The model under review builds one solid part; all positions refer to its coordinate system, in mm. A direction names the side the tool comes from. Give positions to 0.01 mm unless a question says otherwise; leave off trailing zeros. Write each loop counter-clockwise with the first axis right and the second up, starting at its lowest first coordinate (ties: lowest second). Pieces come first, ordered by that corner, then holes. Notation, with made-up numbers: M 11.25,75.25 L 18.25,75.25 A26 ccw 18.25,104.25 Z; hole C 56.5,1.25 d8. An arc over 180 degrees is marked long. Write item = value, one per line. Start each with the question number.
```python
from build123d import *

# Parameters (mm, degrees)
SKETCH_1_R               = 8.75
EXTRUDE_1_DEPTH          = 1
EXTRUDE_2_DEPTH          = 1
SKETCH_3_R               = 2.5
CUT_EXTRUDE_1_DEPTH      = 15.091220671
PATTERN_CIRCULAR_1_COUNT = 20
FILLET_1_R               = 0.25


with BuildPart() as part:
    # 草图1 → 凸台-拉伸1 (new body)
    with BuildSketch(Plane(origin=(0, 0, 0), x_dir=(1, 0, 0), z_dir=(0, 1, 0))):
        with Locations(Location((0, 0, 0), (0, 0, 270))):
            Circle(SKETCH_1_R)
    extrude(amount=-EXTRUDE_1_DEPTH)

    # 草图2 → 凸台-拉伸2 (add)
    with BuildSketch(Plane(origin=(0, 0, 0), x_dir=(1, 0, 0), z_dir=(0, 1, 0))):
        with BuildLine():
            Line((-0.765280386, -10.175), (-0.65625, -8.72535592))
            ThreePointArc((-0.65625, -8.72535592), (0, -8.75), (0.65625, -8.72535592))
            Line((0.65625, -8.72535592), (0.765280386, -10.175))
            ThreePointArc((0.765280386, -10.175), (0, -11), (-0.765280386, -10.175))
        make_face()
    extrude_2 = extrude(amount=-EXTRUDE_2_DEPTH)

    # 草图3 → 切除-拉伸1 (cut, through all)
    with BuildSketch(Plane(origin=(0, 0, 0), x_dir=(1, 0, 0), z_dir=(0, 1, 0))):
        with Locations(Location((0, 0, 0), (0, 0, 270))):
            Circle(SKETCH_3_R)
    extrude(amount=-CUT_EXTRUDE_1_DEPTH, mode=Mode.SUBTRACT)

    # 阵列(圆周)1: 凸台-拉伸2 ×20 about axis
    pattern_circular_1_axis = Axis((0, 0, 0), (0, 1, 0))
    for i in range(1, PATTERN_CIRCULAR_1_COUNT):
        add(extrude_2.rotate(pattern_circular_1_axis, i * 360 / PATTERN_CIRCULAR_1_COUNT))

    # 圆角1
    fillet_1_edges = [part.edges().sort_by_distance(p)[0] for p in [
        (3.3204141, -0.5, -8.095514203),
        (2.072152423, -0.5, -8.501099008),
        (0.65625, -0.5, -8.72535592),
        (-0.65625, -0.5, -8.72535592),
        (-2.072152423, -0.5, -8.501099008),
        (-3.3204141, -0.5, -8.095514203),
        (-4.597718128, -0.5, -7.444695293),
        (-5.659552934, -0.5, -6.67322715),
        (-6.67322715, -0.5, -5.659552934),
        (-7.444695293, -0.5, -4.597718128),
        (-8.095514203, -0.5, -3.3204141),
        (-8.501099008, -0.5, -2.072152423),
        (-8.72535592, -0.5, -0.65625),
        (-8.72535592, -0.5, 0.65625),
        (-8.501099008, -0.5, 2.072152423),
        (-8.095514203, -0.5, 3.3204141),
        (-7.444695293, -0.5, 4.597718128),
        (-6.67322715, -0.5, 5.659552934),
        (-5.659552934, -0.5, 6.67322715),
        (-4.597718128, -0.5, 7.444695293),
        (-3.3204141, -0.5, 8.095514203),
        (-2.072152423, -0.5, 8.501099008),
        (2.072152423, -0.5, 8.501099008),
        (3.3204141, -0.5, 8.095514203),
        (4.597718128, -0.5, 7.444695293),
        (5.659552934, -0.5, 6.67322715),
        (6.67322715, -0.5, 5.659552934),
        (7.444695293, -0.5, 4.597718128),
        (8.095514203, -0.5, 3.3204141),
        (8.501099008, -0.5, 2.072152423),
        (8.72535592, -0.5, 0.65625),
        (8.72535592, -0.5, -0.65625),
        (-0.65625, -0.5, 8.72535592),
        (0.65625, -0.5, 8.72535592),
        (8.501099008, -0.5, -2.072152423),
        (8.095514203, -0.5, -3.3204141),
        (7.444695293, -0.5, -4.597718128),
        (6.67322715, -0.5, -5.659552934),
        (5.659552934, -0.5, -6.67322715),
        (4.597718128, -0.5, -7.444695293),
    ]]
    fillet(fillet_1_edges, radius=FILLET_1_R)


solid = part.part
```
Item 1: We need section D-D, the plane x = 5. Write out the cut boundary in (y, z), and give its area (3 significant figures).
Item 2: For faces 5 (the flat face through (5.04, -0.49, -8.16)), 6 (the flat face through (9.32, -0.49, 2.27)), 7 (the flat face through (-9.58, -0.49, -0.72)), 8 (the flat face through (-2.27, -0.49, 9.32)), list the 3-axis set-ups (+Z, -Z, +X, -X, +Y, -Y) from which the entire face can be reached by the end or side of a thin tool; tool diameter is ignored.
Item 3: We need section A-A, the plane z = 0. Write out the cut boundary in (x, y).
Item 4: We need section C-C, the plane z = 2.75. Write out the cut boundary in (x, y), and give its area (3 significant figures).
Item 5: We need section B-B, the plane x = 0. Write out the cut boundary in (y, z), and give its area (3 significant figures).
Item 6: To check wall thickness, follow probe 1 along Z at (x, y) = (-8.25, -0.35); probe 2 along Z at (x, y) = (6.5, -0.3); probe 3 along X at (y, z) = (-0.3, 8.5). State the ranges of each line that lie inside material, in increasing order. Write a range as [from, to].
Item 7: The part is to be moulded in two halves that separate along X. For faces 1 (the flat face through (-3.64, -0.49, -8.87)), 2 (the flat face through (-9.32, -0.49, -2.27)), 3 (the flat face through (5.05, -0.49, 8.18)), 4 (the cylindrical face through (8.643, -0.493, -1.362)), say which applies: released by +X, released by -X, zero draft, split by the parting line, or undercut.
Worked out:
q1.outline = M -1,-8.1 L 0,-8.1 L 0,8.1 L -1,8.1 Z
q1.area = 16.2 mm²
q2.face_5 = -Z, +Y, -Y
q2.face_6 = +X, +Y, -Y
q2.face_7 = +Y, -Y
q2.face_8 = +Z, +Y, -Y
q3.outline = M -11,-1 L -2.5,-1 L -2.5,0 L -11,0 Z; M 2.5,-1 L 11,-1 L 11,0 L 2.5,0 Z
q4.outline = M -10.38,-1 L 10.38,-1 L 10.38,0 L -10.38,0 Z
q4.area = 20.8 mm²
q5.outline = M -1,-11 L 0,-11 L 0,-2.5 L -1,-2.5 Z; M -1,2.5 L 0,2.5 L 0,11 L -1,11 Z
q5.area = 17.0 mm²
q6.probe_1 = [-6.78, -5.1], [-3.4, 3.4], [5.1, 6.78]
q6.probe_2 = [-8.87, -7.66], [-5.86, 5.86], [7.66, 8.87]
q6.probe_3 = [-6.75, -5.25], [-3.49, 3.49], [5.25, 6.75]
q7.face_1 = undercut
q7.face_2 = released by -X
q7.face_3 = undercut
q7.face_4 = released by +X
